The listing builds one solid part. Answer for the finished solid, in the listing's coordinates (mm). A direction names the side the tool comes from. Coordinates: 2 decimals unless noted, no trailing zeros. Order: outer loops, then holes, each group sorted by start corner. A loop starts at its lowest first (then second) coordinate and runs counter-clockwise, first axis right, second up. Notation, with made-up numbers: (-7, 49.25) - (43, 49.25) arc R7 ccw to (43, 57.25) - close; hole circle Ø8 at (18, 33.25). An arc over 180 degrees is marked (long way). Use a Markdown table: item, result. Add a question column.
Item 1: The part is cut by section C-C, the plane z = -7.5. Give the vertices of the cut face in (x, y).
Item 2: The part is cut by section B-B, the plane y = 20.5. Give the vertices of the cut face in (x, z), then the cut area to 3 significant figures.
Item 3: Find the intervals of material crossed by line 1 along X through (y, z) = (33.5, 14.5); line 2 along X through (y, z) = (20.5, -2); line 3 along Y through (x, z) = (4.5, -17.5), in increasing order.
Item 4: For faces 1 (the cylindrical face through (62.255, 22.343, 0.542)), 2 (the cylindrical face through (1, 48, -21)), determine the directions among +Z, -Z, +X, -X, +Y, -Y from which every point of the face is accessible in a straight line to the end or side of a thin tool.
Item 5: The part is cut by section A-A, the plane z = 0. Give the vertices of the cut face in (x, y), then the cut area to 4 significant figures.
Item 6: The part is cut by section D-D, the plane x = 54. Give the vertices of the cut face in (y, z), then the cut area to 3 significant figures.
Item 7: A flat-ended cylindrical pin translates along its axis: P1, Ø2, axis at y = 15, z = 13.5, coming from the +X side. Find the tip coordinate at first contact, or state that the pin passes through.
from build123d import *

# Parameters (mm, degrees)
SKETCH1_W           = 74
SKETCH1_H           = 44
BOSS_EXTRUDE1_DEPTH = 50
SKETCH2_R           = 12.5
BOSS_EXTRUDE2_DEPTH = 8
SKETCH3_R           = 2.5
BOSS_EXTRUDE3_DEPTH = 35
FILLET1_R           = 5


with BuildPart() as part:
    # Sketch1 → Boss-Extrude1 (new body)
    with BuildSketch(Plane(origin=(0, 0, 0), x_dir=(1, 0, 0), z_dir=(0, 1, 0))):
        Rectangle(SKETCH1_W, SKETCH1_H)
    extrude(amount=BOSS_EXTRUDE1_DEPTH)

    # Sketch2 → Boss-Extrude2 (add)
    with BuildSketch(Plane(origin=(37, 0, 0), x_dir=(0, 0, -1), z_dir=(1, 0, 0))):
        with Locations((0, 25)):
            Circle(SKETCH2_R)
    extrude(amount=BOSS_EXTRUDE2_DEPTH)

    # Sketch3 → Boss-Extrude3 (add)
    with BuildSketch(Plane(origin=(45, 0, 0), x_dir=(0, 0, -1), z_dir=(1, 0, 0))):
        with Locations((0, 24.783973011)):
            Circle(SKETCH3_R)
    extrude(amount=BOSS_EXTRUDE3_DEPTH)

    # Fillet1
    fillet1_edges = [part.edges().sort_by_distance(p)[0] for p in [
        (0, 50, 22),
        (0, 0, 22),
        (0, 0, -22),
        (0, 50, -22),
    ]]
    fillet(fillet1_edges, radius=FILLET1_R)


solid = part.part
Solution:
| question | item | result |
|---|---|---|
| 1 | outline | (-37, 0) - (37, 0) - (37, 15) - (45, 15) - (45, 35) - (37, 35) - (37, 50) - (-37, 50) - close |
| 2 | outline | (-37, -22) - (37, -22) - (37, -11.66) - (45, -11.66) - (45, 11.66) - (37, 11.66) - (37, 22) - (-37, 22) - close |
| 2 | area | 3,440 mm2 |
| 3 | line 1 | x = -37 to 37 |
| 3 | line 2 | x = -37 to 45 |
| 3 | line 3 | y = 0.03 to 49.97 |
| 4 | face 1 | +X |
| 4 | face 2 | -Z, +X, -X, +Y |
| 5 | outline | (-37, 0) - (37, 0) - (37, 12.5) - (45, 12.5) - (45, 22.28) - (80, 22.28) - (80, 27.28) - (45, 27.28) - (45, 37.5) - (37, 37.5) - (37, 50) - (-37, 50) - close |
| 5 | area | 4,075 mm2 |
| 6 | outline | circle Ø5 at (24.78, 0) |
| 6 | area | 19.6 mm2 |
| 7 | P1 | stops at x = 37 |
